```python
from build123d import *

# Parameters (mm, degrees)
SKETCH_1_R      = 3
EXTRUDE_1_DEPTH = 4
CHAMFER_1_SIZE  = 6


with BuildPart() as part:
    # 草图1 → 凸台-拉伸1 (new body)
    with BuildSketch(Plane.XY):
        Polygon((-10, 25), (-1.694756853, 32.21269272), (0.921035956, 30.743806073), (0.186592632, 29.435909669), (8.905901995, 24.539620846), (9.640345319, 25.84751725), (14, 23.399372839), (14, 9.572691833), (12, 9.572691833), (12, 6.915051809), (8, 6.915051809), (8, 0), (0, 0), (0, 7), (-4, 7), (-4, 13), (-10, 13), align=None)
        with Locations((-5, 22)):
            Circle(SKETCH_1_R, mode=Mode.SUBTRACT)
        with Locations((4, 17)):
            Circle(SKETCH_1_R, mode=Mode.SUBTRACT)
    extrude(amount=EXTRUDE_1_DEPTH)

    # 倒角1
    chamfer_1_edges = [part.edges().sort_by_distance(p)[0] for p in [
        (-4, 13, 2),
    ]]
    chamfer(chamfer_1_edges, length=CHAMFER_1_SIZE - 0.0001)  # a hair under: the kernel refuses the full size


solid = part.part
```
Read the model definition and answer for the solid it produces. Units are mm, in the model's axes. A direction names the side the tool comes from. Give positions to 0.01 mm unless a question says otherwise; leave off trailing zeros. Order: outer loops, then holes, each group sorted by start corner. A loop starts at its lowest first (then second) coordinate and runs counter-clockwise, first axis right, second up. Notation, with made-up numbers: (-2.5, -13.5) -> (3.5, -13.5) arc R21 cw to (3.5, -1.5) -> close; hole circle Ø4 at (44, -11). An arc over 180 degrees is marked (long way). One line per item, written item: value. Start each with the question number.
(1) The part is cut by section C-C (x = 4.25). Determine the outline of the cut face in (y, z).
(2) A tool of negligible diameter and unlimited length cuts with its end or side. For faces 1 (the flat face through (-2, 7, 2)), 2 (the flat face through (-5.906, 28.556, 1.972)), 3 (the flat face through (8, 4, 2)), 4 (the flat face through (0.56, 30.1, 1.97)), from which of +Z, -Z, +X, -X, +Y, -Y can it reach the whole face along a straight path? Write none if from no direction.
(3) The part is cut by section A-A (y = 22). Determine the outline of the cut face in (x, z), and give its area (3 significant figures).
(4) The part is cut by section B-B (z = 2.95). State how many separate pieces and enclosed holes the cut face has, and give its area (3 significant figures).
(5) Flat-ended cylindrical pins translate along their axes: P1, Ø1, axis at x = 13, z = 2.5, coming from the -Y side; P2, Ø1.2, axis at x = -1, z = 2.5, coming from the -Y side; P3, Ø5, axis at x = 4, y = 17, coming from the +Z side; P4, Ø1.2, axis at y = 4.5, z = 2.5, coming from the -X side. Find the tip coordinate at first contact, or state that the pin passes through.
(6) The part is cut by section D-D (x = 10.75). Determine the outline of the cut face in (y, z), and give its area (3 significant figures).
(7) Straight lines are drawn through the part: L1, parallel to X at y = 15, z = 3.5; L2, parallel to X at y = 20.5, z = 2.15; L3, parallel to Y at x = 4, z = 2.95. For each, find the intervals that lie inside material, in ascending order.
(8) For a pull along X with two mould halves and no side action, classify faces 5 (the flat face through (-7, 10, 2)), 6 (the flat face through (9.268, 25.184, 1.972)), 7 (the flat face through (0, 16, 0)) as released by +X, released by -X, zero draft, split by the parting line, or undercut.
Taken from the geometry:
1. outline: (0, 0) -> (14.01, 0) -> (14.01, 4) -> (0, 4) -> close; (19.99, 0) -> (27.15, 0) -> (27.15, 4) -> (19.99, 4) -> close
2. face 1: +Z, -Z, -X, -Y
2. face 2: +Z, -Z, -X, +Y
2. face 3: +Z, -Z, +X, -Y
2. face 4: +Z, -Z, +X
3. outline: (-10, 0) -> (-8, 0) -> (-8, 4) -> (-10, 4) -> close; (-2, 0) -> (14, 0) -> (14, 4) -> (-2, 4) -> close
3. area: 72.0 mm^2
4. separate pieces: 1
4. enclosed holes: 2
4. area: 468 mm^2
5. P1: y = 9.57
5. P2: y = 7
5. P3: through
5. P4: x = 0
6. outline: (6.92, 0) -> (25.22, 0) -> (25.22, 4) -> (6.92, 4) -> close
6. area: 73.2 mm^2
7. L1: -10 to 1.76, 6.24 to 14
7. L2: -10 to -7.6, -2.4 to 14
7. L3: 0 to 14, 20 to 27.29
8. face 5: released by -X
8. face 6: undercut
8. face 7: zero draft
